Read the model definition and answer for the solid it produces. Units are mm, in the model's axes. Round coordinates to 2 decimals unless told otherwise and drop trailing zeros. Write each loop counter-clockwise with the first axis right and the second up, starting at its lowest first coordinate (ties: lowest second). Pieces come first, ordered by that corner, then holes. Notation, with made-up numbers: (8, 14) -> (51, 14) arc R13 cw to (51, 24) -> close; hole circle Ø10 at (-27.75, -33.75). An arc over 180 degrees is marked (long way). Return JSON: item names as keys, results as strings.
Autodesk Inventor part; units mm, degrees
ref_plane "XZ Plane" through (0, 0, 0) normal (0, 1, 0) x (-1, 0, 0)
sketch "Sketch1" plane through (0, 0, 0) normal (0, 1, 0) x (-1, 0, 0)
  line L0 (-12, 14) -> (12, 14) construction
  line L1 (14, 12) -> (14, -12) construction
  line L2 (12, -14) -> (-12, -14) construction
  line L3 (-14, -12) -> (-14, 12) construction
  line L4 (-14, 14) -> (14, -14) construction
  line L5 (14, 14) -> (-14, -14) construction
  arc A0 (14, 12) -> (12, 14) centre (12, 12) ccw construction
  arc A1 (12, -14) -> (14, -12) centre (12, -12) ccw construction
  arc A2 (-14, -12) -> (-12, -14) centre (-12, -12) ccw construction
  arc A3 (-12, 14) -> (-14, 12) centre (-12, 12) ccw construction
  line L6 (-12, -15) -> (12, -15)
  arc A4 (12, -15) -> (15, -12) centre (12, -12) ccw
  line L7 (15, -12) -> (15, 12)
  arc A5 (15, 12) -> (12, 15) centre (12, 12) ccw
  line L8 (12, 15) -> (-12, 15)
  arc A6 (-12, 15) -> (-15, 12) centre (-12, 12) ccw
  line L9 (-15, 12) -> (-15, -12)
  arc A7 (-15, -12) -> (-12, -15) centre (-12, -12) ccw
  line L10 (13, -12) -> (13, 12)
  arc A8 (13, 12) -> (12, 13) centre (12, 12) ccw
  line L11 (12, 13) -> (-12, 13)
  arc A9 (-12, 13) -> (-13, 12) centre (-12, 12) ccw
  line L12 (-13, 12) -> (-13, -12)
  arc A10 (-13, -12) -> (-12, -13) centre (-12, -12) ccw
  line L13 (-12, -13) -> (12, -13)
  arc A11 (12, -13) -> (13, -12) centre (12, -12) ccw
  point P0 (0, 0)
  point P1 (0, 0)
  point P2 (0, 0)
  dimension "d10" = 2
  dimension "depth" = 30
  dimension "width" = 30
  dimension "thickness" = 2
extrude "Extrusion1" add sketch "Sketch1" along normal blind 1680
sketch "Sketch2" plane through (12, 0, -15) normal (0, 0, -1) x (-1, 0, 0)
  line L0 (12, -336) -> (12, 2016) construction
  line L1 (0, 0) -> (24, 0)
  line L2 (0, 1680) -> (24, 1680)
  point P0 (12, 0)
  point P1 (12, 50)
  point P2 (12, 100)
  point P3 (12, 1630)
  point P4 (12, 1580)
  dimension "d16" = 50
  dimension "d17" = 50
  dimension "d18" = 50
  dimension "d20" = 50
hole "Hole1" at (0, 50, -15) at (0, 100, -15) at (0, 1630, -15) at (0, 1580, -15) direction (0, 0, 1) diameter 9 depth 20.2 tip angle 118
equation "\"d10\" = thickness"
properties part number "Przedluzka L1680" material "Steel"
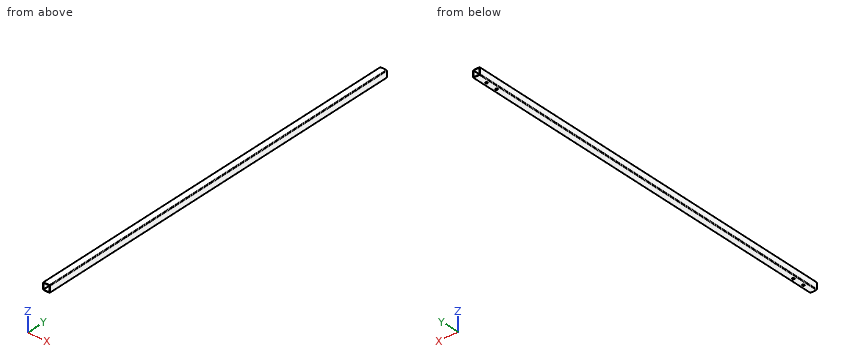
Item 1: Straight lines are drawn through the part: L1, parallel to Y at x = 0, z = -14.3; L2, parallel to X at y = 316, z = -4.25. For each, find the intervals that lie inside material, in ascending order. Write a range as [from, to].
Worked answers:
{"L1": "y = [0, 45.5], [54.5, 95.5], [104.5, 1575.5], [1584.5, 1625.5], [1634.5, 1680]", "L2": "x = [-15, -13], [13, 15]"}
Item 2: Section C-C (y = 366) is taken. Give the vertices of the cut face in (x, z).
Worked answers:
{"outline": "(-15, -12) arc R3 ccw to (-12, -15) -> (12, -15) arc R3 ccw to (15, -12) -> (15, 12) arc R3 ccw to (12, 15) -> (-12, 15) arc R3 ccw to (-15, 12) -> close; hole (-13, -12) arc R1 ccw to (-12, -13) -> (12, -13) arc R1 ccw to (13, -12) -> (13, 12) arc R1 ccw to (12, 13) -> (-12, 13) arc R1 ccw to (-13, 12) -> close"}
Item 3: Section B-B (z = 4.5) is taken. Give the vertices of the cut face in (x, y).
Worked answers:
{"outline": "(-15, 0) -> (-13, 0) -> (-13, 1680) -> (-15, 1680) -> close; (13, 0) -> (15, 0) -> (15, 1680) -> (13, 1680) -> close"}
Item 4: Section A-A (x = 0) is taken. Give the vertices of the cut face in (y, z), then the cut area to 3 significant figures.
Worked answers:
{"outline": "(0, -15) -> (45.5, -15) -> (45.5, -13) -> (0, -13) -> close; (0, 13) -> (1680, 13) -> (1680, 15) -> (0, 15) -> close; (54.5, -15) -> (95.5, -15) -> (95.5, -13) -> (54.5, -13) -> close; (104.5, -15) -> (1575.5, -15) -> (1575.5, -13) -> (104.5, -13) -> close; (1584.5, -15) -> (1625.5, -15) -> (1625.5, -13) -> (1584.5, -13) -> close; (1634.5, -15) -> (1680, -15) -> (1680, -13) -> (1634.5, -13) -> close", "area": "6,650 mm2"}
Item 5: A flat-ended cylindrical pin translates along its axis: pin 1 (7 mm diameter, centred on x = 0, y = 50, fed in from -Z). Find the tip coordinate at first contact, or state that the pin passes through.
Worked answers:
{"pin 1": "stops at z = 13"}
